For this review, take the finished solid that the model builds, in its own axes (mm). A direction names the side the tool comes from. Give positions to 0.01 mm unless a question says otherwise; leave off trailing zeros. Write each loop counter-clockwise with the first axis right and the second up, starting at its lowest first coordinate (ties: lowest second). Pieces come first, ordered by that corner, then holes. Notation, with made-up numbers: (-4, -9) -> (26, -9) arc R21 cw to (26, 13) -> close; hole circle Ø7 at (64.25, -3). An arc over 180 degrees is marked (long way). Write item = value, one per line.
```python
from build123d import *

# Parameters (mm, degrees)
RESSALTO_EXTRUS_O1_DEPTH                             = 4
FILETE1_R                                            = 4
CHANFRO1_SIZE                                        = 1
FURO_DE_DI_METRO_7_0_7_1_D                           = 7
ESCAREADO_PARA_PARAFUSO_COM_CABE_A_ESCAR_D           = 3.4
ESCAREADO_PARA_PARAFUSO_COM_CABE_A_ESCAR_CSINK_D     = 6.3
ESCAREADO_PARA_PARAFUSO_COM_CABE_A_ESCAR_CSINK_ANGLE = 90
BROCA_DE_ROSQUEAR_PARA_TARRAXA_DE_M21_D              = 1.6
BROCA_DE_ROSQUEAR_PARA_TARRAXA_DE_M21_DEPTH          = 8
BROCA_DE_ROSQUEAR_PARA_TARRAXA_DE_M21_TIP            = 0.480688495
FURO_DE_DI_METRO_9_0_9_3_D                           = 9
ESCAREADO_PARA_PARAFUSO_ALLEN_SEXTAVADO_D            = 3.4
ESCAREADO_PARA_PARAFUSO_ALLEN_SEXTAVADO_CSINK_D      = 6.72
ESCAREADO_PARA_PARAFUSO_ALLEN_SEXTAVADO_CSINK_ANGLE  = 90
ESCAREADO_PARA_PARAFUSO_COM_CABE_A_E_2_D             = 3.4
ESCAREADO_PARA_PARAFUSO_COM_CABE_A_E_2_DEPTH         = 4
ESCAREADO_PARA_PARAFUSO_COM_CABE_A_E_2_CSINK_D       = 6.3
ESCAREADO_PARA_PARAFUSO_COM_CABE_A_E_2_CSINK_ANGLE   = 90
ESCAREADO_PARA_PARAFUSO_COM_CABE_A_E_2_TIP           = 1.021463052
ESBO_O12_R                                           = 4.55
CORTE_EXTRUS_O1_DEPTH                                = 3
FURO_DE_DI_METRO_3_5_3_5_1_D                         = 3.5
ESBO_O36_R                                           = 12.5
CORTE_EXTRUS_O4_DEPTH                                = 2


with BuildPart() as part:
    # Esboço1 → Ressalto-extrusão1 (new body)
    with BuildSketch(Plane.XY):
        Polygon((0, 0), (22, 0), (22, 80), (0, 75), align=None)
    extrude(amount=RESSALTO_EXTRUS_O1_DEPTH)

    # Filete1
    filete1_edges = [part.edges().sort_by_distance(p)[0] for p in [
        (0, 75, 2),
        (22, 80, 2),
    ]]
    fillet(filete1_edges, radius=FILETE1_R)

    # Chanfro1
    chanfro1_edges = [part.edges().sort_by_distance(p)[0] for p in [
        (10.113515586, 77.298526269, 0),
        (0, 35.903542878, 0),
        (0.873825208, 74.302487761, 0),
        (20.495402006, 78.115078729, 0),
        (22, 37.494451969, 0),
    ]]
    chamfer(chanfro1_edges, length=CHANFRO1_SIZE)

    # Furo de diâmetro Ø7.0 (7)1 (through all)
    with Locations(Plane(origin=(7.780869527, 38.393713373, 0), x_dir=(-1, 0, 0), z_dir=(0, 0, -1))):
        with Locations((0, 0)):
            Hole(FURO_DE_DI_METRO_7_0_7_1_D / 2)

    # Escareado para parafuso com cabe_a escar (through all)
    with Locations(Plane(origin=(18, 7, 0), x_dir=(-1, 0, 0), z_dir=(0, 0, -1))):
        with Locations((0, 0), (0, 7)):
            CounterSinkHole(ESCAREADO_PARA_PARAFUSO_COM_CABE_A_ESCAR_D / 2, ESCAREADO_PARA_PARAFUSO_COM_CABE_A_ESCAR_CSINK_D / 2, counter_sink_angle=ESCAREADO_PARA_PARAFUSO_COM_CABE_A_ESCAR_CSINK_ANGLE)

    # Broca de rosquear para tarraxa de M21
    with Locations(Plane(origin=(4, 0, 2), x_dir=(0, 0, -1), z_dir=(0, -1, 0))):
        with Locations((0, 0), (0, 8)):
            Hole(BROCA_DE_ROSQUEAR_PARA_TARRAXA_DE_M21_D / 2, depth=BROCA_DE_ROSQUEAR_PARA_TARRAXA_DE_M21_DEPTH)
            with Locations((0, 0, -(BROCA_DE_ROSQUEAR_PARA_TARRAXA_DE_M21_DEPTH + BROCA_DE_ROSQUEAR_PARA_TARRAXA_DE_M21_TIP / 2))):  # 118° drill point
                Cone(0, BROCA_DE_ROSQUEAR_PARA_TARRAXA_DE_M21_D / 2, BROCA_DE_ROSQUEAR_PARA_TARRAXA_DE_M21_TIP, mode=Mode.SUBTRACT)

    # Furo de diâmetro Ø9.0 (9)3 (through all)
    with Locations(Plane(origin=(7.780869527, 60.893713373, 0), x_dir=(-1, 0, 0), z_dir=(0, 0, -1))):
        with Locations((0, 0)):
            Hole(FURO_DE_DI_METRO_9_0_9_3_D / 2)

    # Escareado para parafuso Allen sextavado escareado de M31 (through all)
    with Locations(Plane(origin=(14.368851738, 55.36573993, 0), x_dir=(-1, 0, 0), z_dir=(0, 0, -1))):
        with Locations((0, 0), (13.175964422, 11.055946886)):
            CounterSinkHole(ESCAREADO_PARA_PARAFUSO_ALLEN_SEXTAVADO_D / 2, ESCAREADO_PARA_PARAFUSO_ALLEN_SEXTAVADO_CSINK_D / 2, counter_sink_angle=ESCAREADO_PARA_PARAFUSO_ALLEN_SEXTAVADO_CSINK_ANGLE)

    # Escareado para parafuso com cabe_a e 2
    with Locations(Plane(origin=(18, 30, 0), x_dir=(-1, 0, 0), z_dir=(0, 0, -1))):
        with Locations((0, 0)):
            CounterSinkHole(ESCAREADO_PARA_PARAFUSO_COM_CABE_A_E_2_D / 2, ESCAREADO_PARA_PARAFUSO_COM_CABE_A_E_2_CSINK_D / 2, depth=ESCAREADO_PARA_PARAFUSO_COM_CABE_A_E_2_DEPTH, counter_sink_angle=ESCAREADO_PARA_PARAFUSO_COM_CABE_A_E_2_CSINK_ANGLE)
            with Locations((0, 0, -(ESCAREADO_PARA_PARAFUSO_COM_CABE_A_E_2_DEPTH + ESCAREADO_PARA_PARAFUSO_COM_CABE_A_E_2_TIP / 2))):  # 118° drill point
                Cone(0, ESCAREADO_PARA_PARAFUSO_COM_CABE_A_E_2_D / 2, ESCAREADO_PARA_PARAFUSO_COM_CABE_A_E_2_TIP, mode=Mode.SUBTRACT)

    # Esboço12 → Corte-extrusão1 (cut)
    with BuildSketch(Plane.XY.offset(4)):
        with Locations((7.780869527, 38.393713373)):
            Circle(ESBO_O12_R)
    extrude(amount=-CORTE_EXTRUS_O1_DEPTH, mode=Mode.SUBTRACT)

    # Furo de diâmetro Ø3.5 (3.5)1 (through all)
    with Locations(Plane(origin=(3, 14, 0), x_dir=(-1, 0, 0), z_dir=(0, 0, -1))):
        with Locations((0, 0)):
            Hole(FURO_DE_DI_METRO_3_5_3_5_1_D / 2)

    # Esboço36 → Corte-extrusão4 (cut)
    with BuildSketch(Plane.XY.offset(4)):
        with Locations((7.780869527, 60.893713373)):
            Circle(ESBO_O36_R)
    extrude(amount=-CORTE_EXTRUS_O4_DEPTH, mode=Mode.SUBTRACT)


solid = part.part
```
(1) Take a section at B-B (x = 7.25). Write out the cut boundary in (y, z) (3 decimals), plus the area to 3 significant figures.
Answers below:
outline = (0, 0) -> (34.934, 0) -> (34.934, 1) -> (33.875, 1) -> (33.875, 4) -> (0, 4) -> close; (41.853, 0) -> (56.425, 0) -> (56.425, 2) -> (48.405, 2) -> (48.405, 4) -> (42.913, 4) -> (42.913, 1) -> (41.853, 1) -> close; (65.362, 0) -> (75.622, 0) -> (76.648, 1) -> (76.648, 4) -> (73.382, 4) -> (73.382, 2) -> (65.362, 2) -> close
area = 204 mm^2
(2) Take a section at A-A (y = 7). Write out the cut boundary in (x, z) (3 decimals), plus the area to 3 significant figures.
Answers below:
outline = (0, 1) -> (1, 0) -> (14.85, 0) -> (16.3, 1.45) -> (16.3, 4) -> (0, 4) -> close; (19.7, 1.45) -> (21.075, 0.075) -> (22, 1) -> (22, 4) -> (19.7, 4) -> close; hole circle Ø1.6 at (4, 2); hole circle Ø1.6 at (12, 2)
area = 67.3 mm^2
(3) The part is to be moulded in two halves that separate along X. For faces 3 (the face through (11, 0, 2)), 4 (the face through (7.189, 42.905, 2.521)), 5 (the face through (10.21, 77.32, 2.48)), say which applies: released by +X, released by -X, zero draft, split by the parting line, or undercut.
Answers below:
face_3 = zero draft
face_4 = undercut
face_5 = released by -X
(4) For pin 1 (1.5 mm diameter, centred on x = 3, z = 2, fed in from +Y); pin 2 (2 mm diameter, centred on x = 18, y = 30, fed in from +Z); pin 3 (8 mm diameter, centred on x = 5.5, y = 67.5, fed in from +Z); pin 4 (2 mm diameter, centred on x = 12, z = 2, fed in from +Y), all flat-tipped, find the tip position at first contact; note any pin that passes through.
Answers below:
pin_1 = 75.85
pin_2 = through
pin_3 = 2
pin_4 = 77.95
(5) To check wall thickness, follow probe 1 along X at (y, z) = (6.5, 2.2); probe 2 along Y at (x, z) = (15.5, 0.2); probe 3 along Y at (x, z) = (18, 2.1). State the ranges of each line that lie inside material, in increasing order.
Answers below:
probe_1 = 0 to 3.23, 4.77 to 11.23, 12.77 to 16.38, 19.62 to 22
probe_2 = 0 to 5.43, 8.57 to 12.43, 15.57 to 28.43, 31.57 to 52.42, 58.32 to 77.7
probe_3 = 0 to 5.3, 8.7 to 12.3, 15.7 to 28.3, 31.7 to 53.7, 68.09 to 78.99
(6) Take a section at C-C (y = 30). Write out the cut boundary in (x, z) (3 decimals), plus the area to 3 significant figures.
Answers below:
outline = (0, 1) -> (1, 0) -> (14.85, 0) -> (16.3, 1.45) -> (16.3, 4) -> (0, 4) -> close; (19.7, 1.45) -> (21.075, 0.075) -> (22, 1) -> (22, 4) -> (19.7, 4) -> close
area = 71.3 mm^2
(7) Tool access review of faces 1 (the face through (3.29, 4.06, 2.37)), 2 (the face through (2.772, 15.735, 2.028)): name each direction out of +Z, -Z, +X, -X, +Y, -Y from which nothing blocks a thin tool from reaching the whole face with its end or side.
Answers below:
face_1 = -Y
face_2 = +Z, -Z
